Autodesk Inventor part; units mm, degrees
ref_plane "YZ Plane" through (0, 0, 0) normal (1, 0, 0) x (0, 1, 0)
ref_plane "XZ Plane" through (0, 0, 0) normal (0, 1, 0) x (-1, 0, 0)
ref_plane "XY Plane" through (0, 0, 0) normal (0, 0, 1) x (1, 0, 0)
sketch "Sketch1" plane through (0, 0, 0) normal (0, 0, 1) x (1, 0, 0)
  arc A0 (-50.5454, 57.15) -> (50.5454, 57.15) centre (0, 88.9) ccw
  line L0 (-50.5454, 57.15) -> (-101.6, 57.15)
  line L1 (-101.6, 57.15) -> (-101.6, 0)
  line L2 (-101.6, 0) -> (101.6, 0)
  line L3 (101.6, 0) -> (101.6, 57.15)
  line L4 (101.6, 57.15) -> (50.5454, 57.15)
  line L5 (-142.24, 0) -> (142.24, 0)
  line L6 (0, 57.6383) -> (0, -27.9062) construction
  line L7 (0, -51.2675) -> (0, 112.2612)
  point P0 (0, 0)
  dimension "d32" = 57.15
  dimension "d33" = 59.69
  dimension "d63" = 88.9
  dimension "d64" = 203.2
  dimension "d65" = 101.6
extrude "Extrusion1" add sketch "Sketch1" along normal mid plane 25.4
sketch "Sketch2" plane through (-101.6, 57.15, 12.7) normal (0, 1, 0) x (1, 0, 0)
  line L0 (51.0546, 25.4) -> (51.0546, 0)
  line L1 (51.0546, 0) -> (0, 0)
  line L2 (152.1454, 25.4) -> (152.1454, 0)
  line L3 (203.2, 0) -> (152.1454, 0)
  line L4 (203.2, 25.4) -> (203.2, 0)
  line L5 (0, 0) -> (0, 25.4)
  point P0 (101.6, 12.7)
  point P1 (31.75, 12.7)
  point P2 (171.45, 12.7)
  dimension "d16" = 12.7
  dimension "d18" = 12.7
  dimension "d19" = 31.75
  dimension "d20" = 31.75
hole "Hole1" at (-69.85, 57.15, 0) at (69.85, 57.15, 0) direction (0, -1, 0) diameter 6.7564 end through all
sketch "Sketch4" plane through (0, 0, 12.7) normal (0, 0, 1) x (1, 0, 0)
  line L0 (-46.4578, 51.4224) -> (-59.9282, 37.9521)
  line L1 (-59.9282, 37.9521) -> (-50.9479, 28.9718)
  line L2 (-50.9479, 28.9718) -> (-37.4776, 42.4422)
  line L3 (-37.4776, 42.4422) -> (-46.4578, 51.4224)
  line L4 (37.4776, 42.4422) -> (50.9479, 28.9718)
  line L5 (50.9479, 28.9718) -> (59.9282, 37.9521)
  line L6 (59.9282, 37.9521) -> (46.4578, 51.4224)
  line L7 (46.4578, 51.4224) -> (37.4776, 42.4422)
  line L8 (0, 53.9269) -> (0, 0) construction
  line L9 (-101.6, 0) -> (101.6, 0)
  arc A0 (-50.5454, 57.15) -> (50.5454, 57.15) centre (0, 88.9) ccw
  line L10 (34.6064, 54.2936) -> (52.2131, 36.6869) construction
  line L11 (-58.7882, 30.1118) -> (-24.955, 63.945) construction
  point P0 (46.4578, 51.4224)
  point P1 (-46.4578, 51.4224)
  dimension "d35" = 90
  dimension "d36" = 45
  dimension "d38" = 12.7
  dimension "d39" = 12.7
  dimension "d42" = 6.35
  dimension "d43" = 6.35
  dimension "d46" = 19.05
  dimension "d51" = 19.05
extrude "Extrusion2" cut sketch "Sketch4" against normal through all contours A0 L2 L1 L0 | A0 L6 L5 L4
fillet "Fillet2" radius 3.175 4 edges at (-59.9282, 37.9521, 0) (-50.9479, 28.9718, 0) (50.9479, 28.9718, 0) (59.9282, 37.9521, 0)
sketch "Sketch10" plane through (0, 0, 12.7) normal (0, 0, 1) x (1, 0, 0)
  line L0 (88.9, 12.7) -> (-88.9, 12.7) construction
  line L1 (-101.6, 0) -> (101.6, 0)
  point P0 (0, 0)
  dimension "d91" = 177.8
  dimension "d92" = 88.9
  dimension "d93" = 12.7
hole "Hole5" at (88.9, 12.7, 12.7) at (-88.9, 12.7, 12.7) direction (0, 0, -1) diameter 6.7564 end through all
equation "\"d36\" = 0.5 * d35"
equation "\"d42\" = 0.5 * d39"
equation "\"d43\" = 0.5 * d38"
properties part number "ODSY-0007-004" material "Aluminum 6061"
Part model, mm, in its own coordinate system. A direction names the side the tool comes from. Coordinates: 2 decimals unless noted, no trailing zeros. Order: outer loops, then holes, each group sorted by start corner. A loop starts at its lowest first (then second) coordinate and runs counter-clockwise, first axis right, second up.
(1) Slice it at B-B, the plane y = 12.7. Write the cut outline in (x, z), and give its area (3 significant figures).
Check sheet entries:
outline: (-101.6, -12.7) - (-92.28, -12.7) - (-92.28, 12.7) - (-101.6, 12.7) - close; (-85.52, -12.7) - (85.52, -12.7) - (85.52, 12.7) - (-85.52, 12.7) - close; (92.28, -12.7) - (101.6, -12.7) - (101.6, 12.7) - (92.28, 12.7) - close; hole circle Ø6.76 at (-69.85, 0); hole circle Ø6.76 at (69.85, 0)
area: 4,750 mm2
(2) Slice it at A-A, the plane x = -69.85. Write the cut outline in (y, z), and give its area (3 significant figures).
Check sheet entries:
outline: (0, -12.7) - (57.15, -12.7) - (57.15, -3.38) - (0, -3.38) - close; (0, 3.38) - (57.15, 3.38) - (57.15, 12.7) - (0, 12.7) - close
area: 1,070 mm2
(3) Slice it at C-C, the plane y = 33. Write the cut outline in (x, z).
Check sheet entries:
outline: (-101.6, -12.7) - (-54.98, -12.7) - (-54.98, 12.7) - (-101.6, 12.7) - close; (-46.92, -12.7) - (-20.93, -12.7) - (-20.93, 12.7) - (-46.92, 12.7) - close; (20.93, -12.7) - (46.92, -12.7) - (46.92, 12.7) - (20.93, 12.7) - close; (54.98, -12.7) - (101.6, -12.7) - (101.6, 12.7) - (54.98, 12.7) - close; hole circle Ø6.76 at (-69.85, 0); hole circle Ø6.76 at (69.85, 0)
(4) Pull direction Z, two halves, no side cores. Call faces 1 (the face through (66.5, 28.17, -0.44)), 2 (the face through (-1, 23, 12.7)), 3 (the face through (-1, 0, 0)): pulls with the +Z half, pulls with the -Z half, needs draft (parallel to the pull), parting line crosses it, or undercut.
Check sheet entries:
face 1: undercut
face 2: pulls with the +Z half
face 3: needs draft
(5) Probe L1, parallel to X at y = 20, z = 0; L2, parallel to X at y = 12.7, z = 1; L3, parallel to X at y = 41, z = -6. List the from-to ranges inside material, lowest first.
Check sheet entries:
L1: x = -101.6 to -73.23, -66.47 to 66.47, 73.23 to 101.6
L2: x = -101.6 to -92.28, -85.52 to -73.08, -66.62 to 66.62, 73.08 to 85.52, 92.28 to 101.6
L3: x = -101.6 to -56.88, -38.92 to -35.62, 35.62 to 38.92, 56.88 to 101.6
(6) Tool access for faces 4 (the face through (-101.6, 29, 0)), 5 (the face through (43.01, 36.91, 0.18)), 6 (the face through (-48.56, 54.19, -0.18)): list every direction of +Z, -Z, +X, -X, +Y, -Y with a clear straight run to the whole face (end or side of a thin tool).
Check sheet entries:
face 4: +Z, -Z, -X, +Y, -Y
face 5: +Z, -Z
face 6: +Z, -Z, +Y
(7) Pin check, flat tip, straight feed: pin 1 Ø5.5 at (x, z) = (69.85, 0) entering from -Y. Stop position of the tip, or through.
Check sheet entries:
pin 1: passes through
(8) Slice it at D-D, the plane z = 0. Write the cut outline in (x, y) (3 decimals), and give its area (3 significant figures).
Check sheet entries:
outline: (-101.6, 0) - (-73.228, 0) - (-73.228, 57.15) - (-101.6, 57.15) - close; (-66.472, 0) - (66.472, 0) - (66.472, 57.15) - (50.545, 57.15) arc R59.69 cw to (46.458, 51.422) - (57.683, 40.197) arc R3.175 cw to (57.683, 35.707) - (53.193, 31.217) arc R3.175 cw to (48.703, 31.217) - (37.478, 42.442) arc R59.69 cw to (-37.478, 42.442) - (-48.703, 31.217) arc R3.175 cw to (-53.193, 31.217) - (-57.683, 35.707) arc R3.175 cw to (-57.683, 40.197) - (-46.458, 51.422) arc R59.69 cw to (-50.545, 57.15) - (-66.472, 57.15) - close; (73.228, 0) - (101.6, 0) - (101.6, 57.15) - (73.228, 57.15) - close; hole circle Ø6.756 at (-88.9, 12.7); hole circle Ø6.756 at (88.9, 12.7)
area: 8,310 mm2
